Could you check a few things on this model? Use its own coordinates, in mm. Face numbers are marked on the shaded views. A direction names the side the tool comes from. Coordinates: 2 decimals unless noted, no trailing zeros. Loops run counter-clockwise (first coordinate to the right, second up) from the corner with the lowest first, then second, coordinate; pieces in that order, holes last.
1) Imagine slicing it at A-A on z = 7.5. Please give me the cut outline in (x, y), plus the area to 3 significant figures.
2) If I drill on line 1 along Y through (x, z) = (-1, 8); line 2 along Z through (x, y) = (13.5, -22); line 3 along Y through (x, z) = (30, 2), over which ranges is the centre line in solid material (lowest first)?
3) Will these pins go through, and if not, where does the flat tip stop? P1, Ø3, axis at y = 22.5, z = 10.5, coming from the -X side; P2, Ø8, axis at y = 6.5, z = 45.5, coming from the -X side; P3, Ø5.5, axis at x = 30.5, y = 1.5, coming from the -Z side.
4) Imagine slicing it at B-B on x = 0. Give the number of separate pieces and of enclosed holes in the cut face, plus the area to 3 significant figures.
5) For the marked faces 4 and 5, which set-ups out of +Z, -Z, +X, -X, +Y, -Y let a thin tool reach every point of the face, with its end or its side?
6) Thinking about a two-plate mould opening in X: for the marked faces 1, 2 and 3, which applies, released by +X, released by -X, zero draft, split by the parting line, or undercut?
7) Imagine slicing it at C-C on z = 22. Please give me the cut outline in (x, y), plus the area to 3 significant figures.
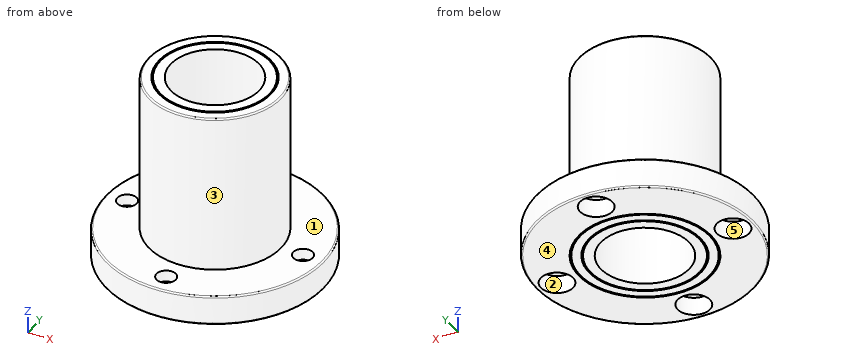
```python
from build123d import *

# Parameters (mm, degrees)
PADR_OCIRCULAR1_COUNT = 4
FILETE1_R             = 0.5


with BuildPart() as part:
    # Esboço1 → Revolução1 (revolve)
    with BuildSketch(Plane(origin=(0, 0, 0), x_dir=(0, 0, -1), z_dir=(1, 0, 0)), mode=Mode.PRIVATE) as revolu_o1_sk:
        Polygon((0, 15), (0, 18.5), (-0.5, 18.5), (-0.5, 19), (0, 19), (0, 22), (-0.5, 22), (-0.5, 22.5), (0, 22.5), (0, 37), (-10, 37), (-10, 22.5), (-64, 22.5), (-64, 19), (-63.5, 19), (-63.5, 18.5), (-64, 18.5), (-64, 15), align=None)
    revolve(revolu_o1_sk.sketch.rotate(Axis((0, 0, 0), (0, 0, 1)), 90), axis=Axis((0, 0, 0), (0, 0, 1)))  # turned: the seam where the file's is

    # Esboço5 → Corte-Revolução1 (revolve, cut)
    with BuildSketch(Plane(origin=(0, 0, 0), x_dir=(0, 0, -1), z_dir=(1, 0, 0)), mode=Mode.PRIVATE) as corte_revolu_o1_sk:
        Polygon((0, 35.5), (-6.1, 35.5), (-6.1, 33.3), (-10, 33.3), (-10, 30), (0, 30), align=None)
    corte_revolu_o1 = revolve(corte_revolu_o1_sk.sketch.rotate(Axis((0, 30, 0), (0, 0, -1)), 180), axis=Axis((0, 30, 0), (0, 0, -1)), mode=Mode.SUBTRACT)  # turned: the seam where the file's is

    # PadrãoCircular1: Corte-Revolução1 ×4 about axis
    padr_ocircular1_axis = Axis((0, 0, 0), (0, 0, 1))
    for i in range(1, PADR_OCIRCULAR1_COUNT):
        add(corte_revolu_o1.rotate(padr_ocircular1_axis, i * 360 / PADR_OCIRCULAR1_COUNT), mode=Mode.SUBTRACT)

    # Filete1
    filete1_edges = [part.edges().sort_by_distance(p)[0] for p in [
        (22.5, 0, 64),
        (37, 0, 10),
        (37, 0, 0),
    ]]
    fillet(filete1_edges, radius=FILETE1_R)


solid = part.part
```
Filled in:
1. outline: circle Ø74 at (0, 0); hole circle Ø6.6 at (-30, 0); hole circle Ø30 at (0, 0); hole circle Ø6.6 at (0, -30); hole circle Ø6.6 at (0, 30); hole circle Ø6.6 at (30, 0)
1. area: 3,460 mm2
2. line 1: y = -36.99 to -33.14, -26.86 to -14.97, 14.97 to 26.86, 33.14 to 36.99
2. line 2: z = 0 to 10
2. line 3: y = -21.66 to -5.5, 5.5 to 21.66
3. P1: stops at x = -30.25
3. P2: stops at x = -22.36
3. P3: stops at z = 6.1
4. separate pieces: 4
4. enclosed holes: 0
4. area: 1,060 mm2
5. face 4: -Z, +X, -X, +Y, -Y
5. face 5: -Z
6. face 1: zero draft
6. face 2: undercut
6. face 3: split by the parting line
7. outline: circle Ø45 at (0, 0); hole circle Ø30 at (0, 0)
7. area: 884 mm2
